Check sheet for the modelled part. Datum: model origin and axes. Units: mm. A direction names the side the tool comes from. Round coordinates to 2 decimals unless told otherwise and drop trailing zeros. Order: outer loops, then holes, each group sorted by start corner. A loop starts at its lowest first (then second) coordinate and runs counter-clockwise, first axis right, second up.
Q1. Scan lines: probe 1 along Y at (x, z) = (0, 0.75); probe 2 along Z at (x, y) = (-5, -3); probe 3 along Z at (x, y) = (8.75, 1.5). Record each from-to range of solid material in increasing order.
Q2. Mould release check, pull along Y, two halves, no side actions. Record for faces 4 (the flat face through (-2, 3.95, -2)), 5 (the flat face through (-2, -3.95, -2)), 6 (the cylindrical face through (1.846, -3.549, -1.451)): +Y half, -Y half, draft (parallel to the pull), parting line (faces both ways), or undercut.
Q3. Cross-section at D-D on x = 4.25. Record the cut outline in (y, z), then the cut area to 3 significant figures.
Q4. Cross-section at A-A on z = 4.5. Record the cut outline in (x, y), then the cut area to 3 significant figures.
Q5. Cross-section at C-C on y = 0. Record the cut outline in (x, z).
Q6. Set-up check for faces 1 (the flat face through (3.95, 2, -2)), 2 (the flat face through (2, 3.95, -2)), 3 (the flat face through (-3.463, -5.794, 4.535)): record each of +Z, -Z, +X, -X, +Y, -Y from which the full face is reachable in a straight line by a thin tool's end or side.
Q7. Depth check by flat-ended pin: P1, Ø1, axis at y = 2.5, z = -3, coming from the -X side; P2, Ø1.7, axis at x = -3, z = -2, coming from the -Y side; P3, Ø1.7, axis at x = -2, z = -1.5, coming from the +Y side; P4, Ø11, axis at x = 2, y = -3.5, coming from the +Z side. Enter the tip coordinate at first touch or a pass-through.
Q8. Cross-section at B-B on x = -3. Record the cut outline in (y, z), then the cut area to 3 significant figures.
from build123d import *

# Parameters (mm, degrees)
F0_R     = 9.5
F1_DEPTH = 7
F3_DEPTH = 5
F4_W     = 7.9
F4_H     = 7.9
F5_DEPTH = 5
F6_R     = 4
F7_DEPTH = 7.001


with BuildPart() as f1:
    # F0 (on Top) → F1 (new body)
    with BuildSketch(Plane.XY):
        Circle(F0_R)
    extrude(amount=F1_DEPTH)

    # F2 (on face) → F3 (cut)
    with BuildSketch(Plane.XY.offset(7)):
        Polygon((-0.054944, -7.794035), (6.72236, -3.944601), (6.777304, 3.849434), (0.054944, 7.794035), (-6.72236, 3.944601), (-6.777304, -3.849434), align=None)
    extrude(amount=-F3_DEPTH, mode=Mode.SUBTRACT)

    # F4 (on face) → F5 (join)
    with BuildSketch(Plane(origin=(0, 0, 0), x_dir=(1, 0, 0), z_dir=(0, 0, -1))):
        Rectangle(F4_W, F4_H)
    extrude(amount=F5_DEPTH)

    # F6 (on face) → F7 (cut, through all)
    with BuildSketch(Plane.XY.offset(2)):
        Circle(F6_R)
    extrude(amount=-F7_DEPTH, mode=Mode.SUBTRACT)


solid = f1.part
Results found:
1. probe 1: y = -9.5 to -4, 4 to 9.5
1. probe 2: z = 0 to 2
1. probe 3: z = 0 to 7
2. face 4: +Y half
2. face 5: -Y half
2. face 6: undercut
3. outline: (-8.5, 0) - (8.5, 0) - (8.5, 7) - (5.33, 7) - (5.33, 2) - (-5.35, 2) - (-5.35, 7) - (-8.5, 7) - close
3. area: 65.5 mm2
4. outline: circle Ø19 at (0, 0); hole (-6.78, -3.85) - (-0.05, -7.79) - (6.72, -3.94) - (6.78, 3.85) - (0.05, 7.79) - (-6.72, 3.94) - close
4. area: 126 mm2
5. outline: (-9.5, 0) - (-4, 0) - (-4, 2) - (-6.75, 2) - (-6.75, 7) - (-9.5, 7) - close; (4, 0) - (9.5, 0) - (9.5, 7) - (6.75, 7) - (6.75, 2) - (4, 2) - close
6. face 1: -Z, +X, +Y, -Y
6. face 2: -Z, +X, -X, +Y
6. face 3: +Z
7. P1: stops at x = -3.95
7. P2: stops at y = -3.95
7. P3: stops at y = 3.95
7. P4: stops at z = 7
8. outline: (-9.01, 0) - (-3.95, 0) - (-3.95, -5) - (-2.65, -5) - (-2.65, 2) - (-6.07, 2) - (-6.07, 7) - (-9.01, 7) - close; (2.65, -5) - (3.95, -5) - (3.95, 0) - (9.01, 0) - (9.01, 7) - (6.06, 7) - (6.06, 2) - (2.65, 2) - close
8. area: 68.0 mm2
